from build123d import *

# Parameters (mm, degrees)
SKETCH_1_W          = 40
SKETCH_1_H          = 20
SKETCH_1_W_2        = 38
SKETCH_1_H_2        = 18
EXTRUDE_1_DEPTH     = 550
SKETCH_4_R          = 1.75
CUT_EXTRUDE_2_DEPTH = 1.5
SKETCH_5_R          = 2.6
CUT_EXTRUDE_3_DEPTH = 1.5
SKETCH_6_R          = 2.5
CUT_EXTRUDE_4_DEPTH = 552.815186453


with BuildPart() as part:
    # 草图1 → 拉伸-薄壁1 (new body)
    with BuildSketch(Plane.XY):
        with Locations((20, -10)):
            Rectangle(SKETCH_1_W, SKETCH_1_H)
        with Locations((20, -10)):
            Rectangle(SKETCH_1_W_2, SKETCH_1_H_2, mode=Mode.SUBTRACT)
    extrude(amount=EXTRUDE_1_DEPTH)

    # 草图4 → 切除-拉伸2 (cut)
    with BuildSketch(Plane.ZY):
        with Locations((539.996387591, -10)):
            Circle(SKETCH_4_R)
        with Locations((10, -10.000000002)):
            Circle(SKETCH_4_R)
    extrude(amount=-CUT_EXTRUDE_2_DEPTH, mode=Mode.SUBTRACT)

    # 草图5 → 切除-拉伸3 (cut)
    with BuildSketch(Plane.ZY):
        with Locations((255, -10)):
            Circle(SKETCH_5_R)
    extrude(amount=-CUT_EXTRUDE_3_DEPTH, mode=Mode.SUBTRACT)

    # 草图6 → 切除-拉伸4 (cut, through all)
    with BuildSketch(Plane(origin=(40, 0, 0), x_dir=(0, 0, -1), z_dir=(1, 0, 0))):
        with Locations((-320, -10)):
            Circle(SKETCH_6_R)
        with Locations((-230, -10)):
            Circle(SKETCH_6_R)
    extrude(amount=-CUT_EXTRUDE_4_DEPTH, mode=Mode.SUBTRACT)


solid = part.part
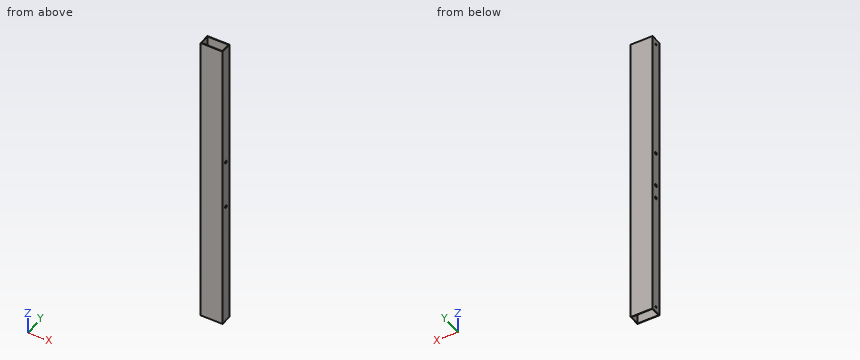
CAD build for the part. Positions are in the model's coordinates, mm. Coordinates: 2 decimals unless noted, no trailing zeros. Loops run counter-clockwise (first coordinate to the right, second up) from the corner with the lowest first, then second, coordinate; pieces in that order, holes last. Notation, with made-up numbers: (87, 12.5) - (142, 12.5) arc R12 ccw to (142, 21.5) - close; hole circle Ø11 at (-13.75, 64.25). An arc over 180 degrees is marked (long way). Use one line per item in the form item = value. Start each with the question number.
1) Flat gauge pins, fed straight in: pin 1 (1 mm diameter, centred on y = -18, z = 282.5, fed in from -X); pin 2 (2 mm diameter, centred on y = -10, z = 10, fed in from -X). Where does each tip first touch, or does it go through?
2) Drill centre lines: L1, parallel to Y at x = 21, z = 265; L2, parallel to X at y = -8, z = 225. Where is each one in solid material? Low to high. Write a range as from..to.
3) Band-saw the part on B-B (x = 22). Give the cut face in (y, z), and give its area (3 significant figures).
4) Band-saw the part on A-A (z = 455.5). Give the cut face in (x, y), and give its area (3 significant figures).
5) Band-saw the part on C-C (y = -4). Give the cut face in (x, z), and give its area (3 significant figures).
Check values:
q1.pin_1 = 0
q1.pin_2 = 39
q2.L1 = -20..-19, -1..0
q2.L2 = 0..1, 39..40
q3.outline = (-20, 0) - (-19, 0) - (-19, 550) - (-20, 550) - close; (-1, 0) - (0, 0) - (0, 550) - (-1, 550) - close
q3.area = 1,100 mm2
q4.outline = (0, -20) - (40, -20) - (40, 0) - (0, 0) - close; hole (1, -19) - (39, -19) - (39, -1) - (1, -1) - close
q4.area = 116 mm2
q5.outline = (0, 0) - (1, 0) - (1, 550) - (0, 550) - close; (39, 0) - (40, 0) - (40, 550) - (39, 550) - close
q5.area = 1,100 mm2
